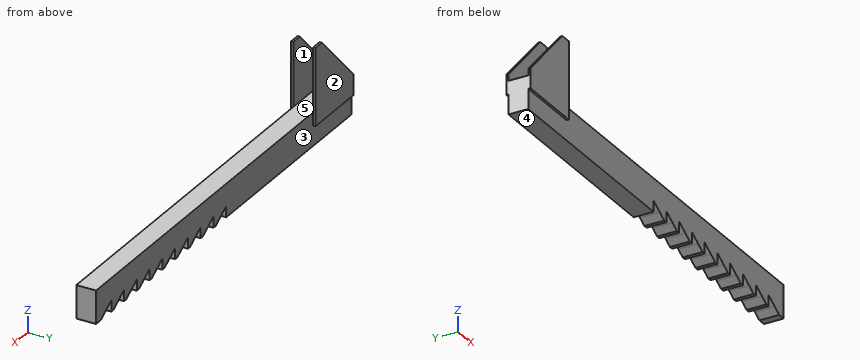
from build123d import *

# Parameters (mm, degrees)
F1_DEPTH = 4.5
F4_DEPTH = 1


with BuildPart() as f1:
    # F0 (on Front) → F1 (new body, symmetric)
    with BuildSketch(Plane.XZ):
        Polygon((-10, 3.8), (-7.132532, 2.079519), (-3.666667, 0), (-3.48962, 0), (-2, 0), (-2, 5), (0, 3.8), (2.867468, 2.079519), (6.333333, 0), (6.51038, 0), (8, 0), (8, 5), (10, 3.8), (12.867468, 2.079519), (16.333333, 0), (16.51038, 0), (18, 0), (18, 5), (20, 3.8), (22.867468, 2.079519), (26.333333, 0), (26.51038, 0), (28, 0), (28, 5), (30, 3.8), (32.867468, 2.079519), (36.333333, 0), (36.51038, 0), (38, 0), (38, 5), (40, 3.8), (42.867468, 2.079519), (46.333333, 0), (46.51038, 0), (48, 0), (48, 5), (50, 3.8), (52.867468, 2.079519), (56.333333, 0), (56.51038, 0), (58, 0), (58, 5), (60, 3.8), (62.867468, 2.079519), (66.333333, 0), (66.51038, 0), (68, 0), (68, 5), (70, 3.8), (72.867468, 2.079519), (76.333333, 0), (76.51038, 0), (78, 0), (78, 5), (80, 3.8), (82.867468, 2.079519), (86.333333, 0), (86.51038, 0), (89.901179, 0.061058), (89.901179, 15), (-110.098821, 15), (-110.098821, 0), (-12, 0), (-12, 5), align=None)
    extrude(amount=F1_DEPTH, both=True)

    # F3 (on offset) → F4 (join)
    with BuildSketch(Plane.XZ.offset(4.5)):
        Polygon((-80.098821, 44), (-85.098821, 44), (-110.098821, 18), (-110.098821, 9), (-80.098821, 9), align=None)
    extrude(amount=F4_DEPTH)

    # F5: F1 across plane


with BuildPart() as f1_1:
    add(f1.part)
    add(f1.part.mirror(Plane.XZ))


solid = f1_1.part
Check sheet for the modelled part. Datum: model origin and axes. Units: mm. Face numbers are marked on the shaded views. A direction names the side the tool comes from. Give positions to 0.01 mm unless a question says otherwise; leave off trailing zeros. Loops run counter-clockwise (first coordinate to the right, second up) from the corner with the lowest first, then second, coordinate; pieces in that order, holes last. Notation, with made-up numbers: M 37,10.5 L 63,10.5 A25 cw 63,29.5 Z; hole C 57,0 d8. An arc over 180 degrees is marked long. Answer as a JSON object with one key per item and string values. Group by question number.
Q1. Access from +Z, -Z, +X, -X, +Y, -Y to the whole of each face (thin tool, end or side, straight path). Record for the marked faces 1 and 2.
Q2. Cross-section at B-B on x = -82. Record the cut outline in (y, z).
Q3. Release check for a two-part mould opening along Z. For the marked faces 3, 4 and 5 record: released by +Z, released by -Z, zero draft, split by the parting line, or undercut.
Q4. Cross-section at C-C on z = 37. Record the cut outline in (x, y).
Q5. Cross-section at A-A on z = 26.5. Record the cut outline in (x, y).
Q6. Cross-section at D-D on x = -43.5. Record the cut outline in (y, z), then the cut area to 3 significant figures.
Q7. Go/stop test with flat-tipped pins: P1, Ø0.8, axis at x = -98, y = 5, coming from the -Z side; P2, Ø0.5, axis at y = 5, z = 18.5, coming from the +X side; P3, Ø4.5, axis at x = -41.5, y = -0.5, coming from the +Z side. Record where each tip stops, or that it passes through.
Q8. Material ranges on line 1 along Y through (x, z) = (-87.5, 40.5); line 2 along Z through (x, y) = (-72.5, 0.25); line 3 along Y through (x, z) = (9, 7.5), recorded low to high. Write a range as [from, to].
Evaluation:
{
 "1": {"face 1": "+Z, +X, -X", "face 2": "+Z, -Z, +X, -X, +Y"},
 "2": {"outline": "M -5.5,9 L -4.5,9 L -4.5,0 L 4.5,0 L 4.5,9 L 5.5,9 L 5.5,44 L 4.5,44 L 4.5,15 L -4.5,15 L -4.5,44 L -5.5,44 Z"},
 "3": {"face 3": "zero draft", "face 4": "released by -Z", "face 5": "released by +Z"},
 "4": {"outline": "M -91.83,-5.5 L -80.1,-5.5 L -80.1,-4.5 L -91.83,-4.5 Z; M -91.83,4.5 L -80.1,4.5 L -80.1,5.5 L -91.83,5.5 Z"},
 "5": {"outline": "M -101.93,-5.5 L -80.1,-5.5 L -80.1,-4.5 L -101.93,-4.5 Z; M -101.93,4.5 L -80.1,4.5 L -80.1,5.5 L -101.93,5.5 Z"},
 "6": {"outline": "M -4.5,0 L 4.5,0 L 4.5,15 L -4.5,15 Z", "area": "135 mm2"},
 "7": {"P1": "stops at z = 9", "P2": "stops at x = -80.1", "P3": "stops at z = 15"},
 "8": {"line 1": "y = [-5.5, -4.5], [4.5, 5.5]", "line 2": "z = [0, 15]", "line 3": "y = [-4.5, 4.5]"}
}
